from build123d import *

# Parameters (mm, degrees)
F3_W         = 27
F3_H         = 27
F4_DEPTH     = 30
F5_T1_DEPTH  = 407
F5_T3_DEPTH  = 443
F5_T5_DEPTH  = 442
F5_T7_DEPTH  = 478
F5_T13_DEPTH = 447
F5_T17_DEPTH = 412
F5_T20_DEPTH = 417
F5_T22_DEPTH = 455
F5_T24_DEPTH = 410
F5_T26_DEPTH = 445
F5_T28_DEPTH = 490
F5_T30_DEPTH = 452
F5_T36_DEPTH = 415
F5_T40_DEPTH = 450
F5_T47_DEPTH = 415
F5_T51_DEPTH = 450


# Not quite as in the source:
# - a fillet or chamfer that OpenCascade refuses, or shapes differently, is made with other operations: its cross-section is extruded or revolved along the edge and cut away or added


with BuildPart() as f2:
    # F2: sweep along a path in F1
    with BuildLine(Plane.XY) as f2_path:
        Line((0, 0), (0, 440))
        Line((0, 440), (-405, 440))
    # F0 (on Front) → F2 (sweep)
    with BuildSketch(Plane.XZ):
        Polygon((38, -2), (38, -25), (40, -25), (40, 0), (0, 0), (0, -350), (27, -350), (27, -376), (29, -376), (29, -348), (2, -348), (2, -2), align=None)
    sweep(path=f2_path.line, transition=Transition.RIGHT)

    # F3 (on face) → F4 (cut)
    with BuildSketch(Plane.XY.offset(-348)):
        with Locations((15.5, 455.5)):
            Rectangle(F3_W, F3_H)
    extrude(amount=-F4_DEPTH, mode=Mode.SUBTRACT)

    # F5: fillet of radius 2 on 15 edges, made by hand

    # F5_s2 → F5_t1 (join)
    with BuildSketch(Plane.YZ.offset(-405)):
        with BuildLine():
            ThreePointArc((442, -346), (442.5857864376, -347.4142135624), (444, -348))
            Line((444, -348), (442, -348))
            Line((442, -348), (442, -346))
        make_face()
        with BuildLine():
            ThreePointArc((465, -350), (466.4142135624, -350.5857864376), (467, -352))
            Line((467, -352), (467, -350))
            Line((467, -350), (465, -350))
        make_face()
        with BuildLine():
            ThreePointArc((444, -2), (442.5857864376, -2.5857864376), (442, -4))
            Line((442, -4), (442, -2))
            Line((442, -2), (444, -2))
        make_face()
    extrude(amount=F5_T1_DEPTH)

    # F5_s4 → F5_t3 (join)
    with BuildSketch(Plane.YZ.offset(-405)):
        with BuildLine():
            ThreePointArc((476, -2), (477.4142135624, -2.5857864376), (478, -4))
            Line((478, -4), (478, -2))
            Line((478, -2), (476, -2))
        make_face()
    extrude(amount=F5_T3_DEPTH)

    # F5_s6 → F5_t5 (join)
    with BuildSketch(Plane.XZ.offset(-442)):
        with BuildLine():
            ThreePointArc((25, -350), (26.4142135624, -350.5857864376), (27, -352))
            Line((27, -352), (27, -350))
            Line((27, -350), (25, -350))
        make_face()
        with BuildLine():
            ThreePointArc((4, -2), (2.5857864376, -2.5857864376), (2, -4))
            Line((2, -4), (2, -2))
            Line((2, -2), (4, -2))
        make_face()
    extrude(amount=F5_T5_DEPTH)

    # F5_s8 → F5_t7 (join)
    with BuildSketch(Plane.XZ.offset(-478)):
        with BuildLine():
            ThreePointArc((38, -4), (37.4142135624, -2.5857864376), (36, -2))
            Line((36, -2), (38, -2))
            Line((38, -2), (38, -4))
        make_face()
    extrude(amount=F5_T7_DEPTH)


with BuildPart() as f5_tool11:
    # F5_s12 → F5_t13 (new body)
    with BuildSketch(Plane.XZ):
        with BuildLine():
            ThreePointArc((4, -2), (2.5857864376, -2.5857864376), (2, -4))
            Line((2, -4), (2, -2))
            Line((2, -2), (4, -2))
        make_face()
    extrude(amount=-F5_T13_DEPTH)

    split(bisect_by=Plane.XZ.offset(-442), keep=Keep.BOTTOM)


with BuildPart() as f5_tool15:
    # F5_s16 → F5_t17 (new body)
    with BuildSketch(Plane.YZ.offset(7)):
        with BuildLine():
            ThreePointArc((444, -2), (442.5857864376, -2.5857864376), (442, -4))
            Line((442, -4), (442, -2))
            Line((442, -2), (444, -2))
        make_face()
    extrude(amount=-F5_T17_DEPTH)

    split(bisect_by=Plane.YZ.offset(2), keep=Keep.TOP)


with BuildPart() as f5_tool11_1:
    add(f5_tool11.part)

    # F5_t19: intersect F5_tool15
    add(f5_tool15.part, mode=Mode.INTERSECT)


with BuildPart() as f2_1:
    add(f2.part)

    # F5_t9: union F5_tool11
    add(f5_tool11_1.part)

    # F5_s21 → F5_t20 (cut)
    with BuildSketch(Plane.YZ.offset(-410)):
        with BuildLine():
            ThreePointArc((467, -348), (468.4142135624, -348.5857864376), (469, -350))
            Line((469, -350), (469, -348))
            Line((469, -348), (467, -348))
        make_face()
    extrude(amount=F5_T20_DEPTH, mode=Mode.SUBTRACT)

    # F5_s23 → F5_t22 (cut)
    with BuildSketch(Plane.YZ.offset(-410)):
        with BuildLine():
            ThreePointArc((480, -2), (479.4142135624, -0.5857864376), (478, 0))
            Line((478, 0), (480, 0))
            Line((480, 0), (480, -2))
        make_face()
    extrude(amount=F5_T22_DEPTH, mode=Mode.SUBTRACT)

    # F5_s25 → F5_t24 (cut)
    with BuildSketch(Plane.YZ.offset(-410)):
        with BuildLine():
            ThreePointArc((440, -2), (440.5857864376, -0.5857864376), (442, 0))
            Line((442, 0), (440, 0))
            Line((440, 0), (440, -2))
        make_face()
        with BuildLine():
            ThreePointArc((440, -348), (440.5857864376, -349.4142135624), (442, -350))
            Line((442, -350), (440, -350))
            Line((440, -350), (440, -348))
        make_face()
    extrude(amount=F5_T24_DEPTH, mode=Mode.SUBTRACT)

    # F5_s27 → F5_t26 (cut)
    with BuildSketch(Plane.XZ.offset(-440)):
        with BuildLine():
            ThreePointArc((0, -2), (0.5857864376, -0.5857864376), (2, 0))
            Line((2, 0), (0, 0))
            Line((0, 0), (0, -2))
        make_face()
        with BuildLine():
            ThreePointArc((2, -350), (0.5857864376, -349.4142135624), (0, -348))
            Line((0, -348), (0, -350))
            Line((0, -350), (2, -350))
        make_face()
    extrude(amount=F5_T26_DEPTH, mode=Mode.SUBTRACT)

    # F5_s29 → F5_t28 (cut)
    with BuildSketch(Plane.XZ.offset(-485)):
        with BuildLine():
            ThreePointArc((38, 0), (39.4142135624, -0.5857864376), (40, -2))
            Line((40, -2), (40, 0))
            Line((40, 0), (38, 0))
        make_face()
    extrude(amount=F5_T28_DEPTH, mode=Mode.SUBTRACT)

    # F5_s31 → F5_t30 (cut)
    with BuildSketch(Plane.XZ.offset(-447)):
        with BuildLine():
            ThreePointArc((27, -348), (28.4142135624, -348.5857864376), (29, -350))
            Line((29, -350), (29, -348))
            Line((29, -348), (27, -348))
        make_face()
    extrude(amount=F5_T30_DEPTH, mode=Mode.SUBTRACT)


with BuildPart() as f5_tool34:
    # F5_s35 → F5_t36 (new body)
    with BuildSketch(Plane.YZ.offset(5)):
        with BuildLine():
            ThreePointArc((440, -2), (440.5857864376, -0.5857864376), (442, 0))
            Line((442, 0), (440, 0))
            Line((440, 0), (440, -2))
        make_face()
    extrude(amount=-F5_T36_DEPTH)

    split(bisect_by=Plane.YZ, keep=Keep.TOP)


with BuildPart() as f5_tool38:
    # F5_s39 → F5_t40 (new body)
    with BuildSketch(Plane.XZ.offset(5)):
        with BuildLine():
            ThreePointArc((0, -2), (0.5857864376, -0.5857864376), (2, 0))
            Line((2, 0), (0, 0))
            Line((0, 0), (0, -2))
        make_face()
    extrude(amount=-F5_T40_DEPTH)

    split(bisect_by=Plane.XZ.offset(-440), keep=Keep.BOTTOM)


with BuildPart() as f5_tool34_1:
    add(f5_tool34.part)

    # F5_t42: intersect F5_tool38
    add(f5_tool38.part, mode=Mode.INTERSECT)


with BuildPart() as f2_2:
    add(f2_1.part)

    # F5_t32: cut F5_tool34
    add(f5_tool34_1.part, mode=Mode.SUBTRACT)


with BuildPart() as f5_tool45:
    # F5_s46 → F5_t47 (new body)
    with BuildSketch(Plane.YZ.offset(5)):
        with BuildLine():
            ThreePointArc((440, -348), (440.5857864376, -349.4142135624), (442, -350))
            Line((442, -350), (440, -350))
            Line((440, -350), (440, -348))
        make_face()
    extrude(amount=-F5_T47_DEPTH)

    split(bisect_by=Plane.YZ, keep=Keep.TOP)


with BuildPart() as f5_tool49:
    # F5_s50 → F5_t51 (new body)
    with BuildSketch(Plane.XZ.offset(5)):
        with BuildLine():
            ThreePointArc((2, -350), (0.5857864376, -349.4142135624), (0, -348))
            Line((0, -348), (0, -350))
            Line((0, -350), (2, -350))
        make_face()
    extrude(amount=-F5_T51_DEPTH)

    split(bisect_by=Plane.XZ.offset(-440), keep=Keep.BOTTOM)


with BuildPart() as f5_tool45_1:
    add(f5_tool45.part)

    # F5_t53: intersect F5_tool49
    add(f5_tool49.part, mode=Mode.INTERSECT)


with BuildPart() as f2_3:
    add(f2_2.part)

    # F5_t43: cut F5_tool45
    add(f5_tool45_1.part, mode=Mode.SUBTRACT)


solid = f2_3.part
Geometry check sheet. Reference: the model listing, model coordinates, mm. A direction names the side the tool comes from. Round coordinates to 2 decimals unless told otherwise and drop trailing zeros. Write each loop counter-clockwise with the first axis right and the second up, starting at its lowest first coordinate (ties: lowest second). Pieces come first, ordered by that corner, then holes.
Item 1: Section check A-A (x = -25). Record the boundary of the cut face in (y, z).
Determined:
outline: (440, -348) arc R2 ccw to (442, -350) - (465, -350) arc R2 cw to (467, -352) - (467, -376) - (469, -376) - (469, -350) arc R2 ccw to (467, -348) - (444, -348) arc R2 cw to (442, -346) - (442, -4) arc R2 cw to (444, -2) - (476, -2) arc R2 cw to (478, -4) - (478, -25) - (480, -25) - (480, -2) arc R2 ccw to (478, 0) - (442, 0) arc R2 ccw to (440, -2) - close
Item 2: Access from +Z, -Z, +X, -X, +Y, -Y to the whole of each face (thin tool, end or side, straight path). Record for faces 1 (the face through (27, 224, -364)), 2 (the face through (29, 224, -363)), 3 (the face through (0, 223, -173)).
Determined:
face 1: -Z, -X, +Y, -Y
face 2: -Z, +X, +Y, -Y
face 3: +Z, -Z, -X, -Y
Item 3: Section check B-B (y = 355). Record the boundary of the cut face in (x, z).
Determined:
outline: (0, -348) arc R2 ccw to (2, -350) - (25, -350) arc R2 cw to (27, -352) - (27, -376) - (29, -376) - (29, -350) arc R2 ccw to (27, -348) - (2, -348) - (2, -4) arc R2 cw to (4, -2) - (36, -2) arc R2 cw to (38, -4) - (38, -25) - (40, -25) - (40, -2) arc R2 ccw to (38, 0) - (2, 0) arc R2 ccw to (0, -2) - close
Item 4: Material ranges on line 1 along Y through (x, z) = (-277.5, -309.5); line 2 along X through (y, z) = (262.5, -288); line 3 along Z through (x, y) = (5, 132.5), recorded low to high.
Determined:
line 1: y = 440 to 442
line 2: x = 0 to 2
line 3: z = -350 to -348, -2 to 0
Item 5: Mould release check, pull along Y, two halves, no side actions. Record for faces 4 (the face through (38, 242, -14)), 5 (the face through (-204, 467, -364)), 6 (the face through (-186, 480, -14)), 7 (the face through (-187, 478, -14)): +Y half, -Y half, draft (parallel to the pull), parting line (faces both ways), or undercut.
Determined:
face 4: draft
face 5: -Y half
face 6: +Y half
face 7: undercut
Item 6: Go/stop test with flat-tipped pins: pin 1 Ø21 at (x, z) = (-117.5, -360) entering from +Y; pin 2 Ø1.5 at (y, z) = (62, -230.5) entering from -X; pin 3 Ø12 at (x, z) = (-107, -194) entering from -Y. Record where each tip stops, or that it passes through.
Determined:
pin 1: stops at y = 469
pin 2: stops at x = 0
pin 3: stops at y = 440
Item 7: Section check C-C (z = -219.5). Record the boundary of the cut face in (x, y).
Determined:
outline: (-405, 440) - (0, 440) - (0, 0) - (2, 0) - (2, 442) - (-405, 442) - close
